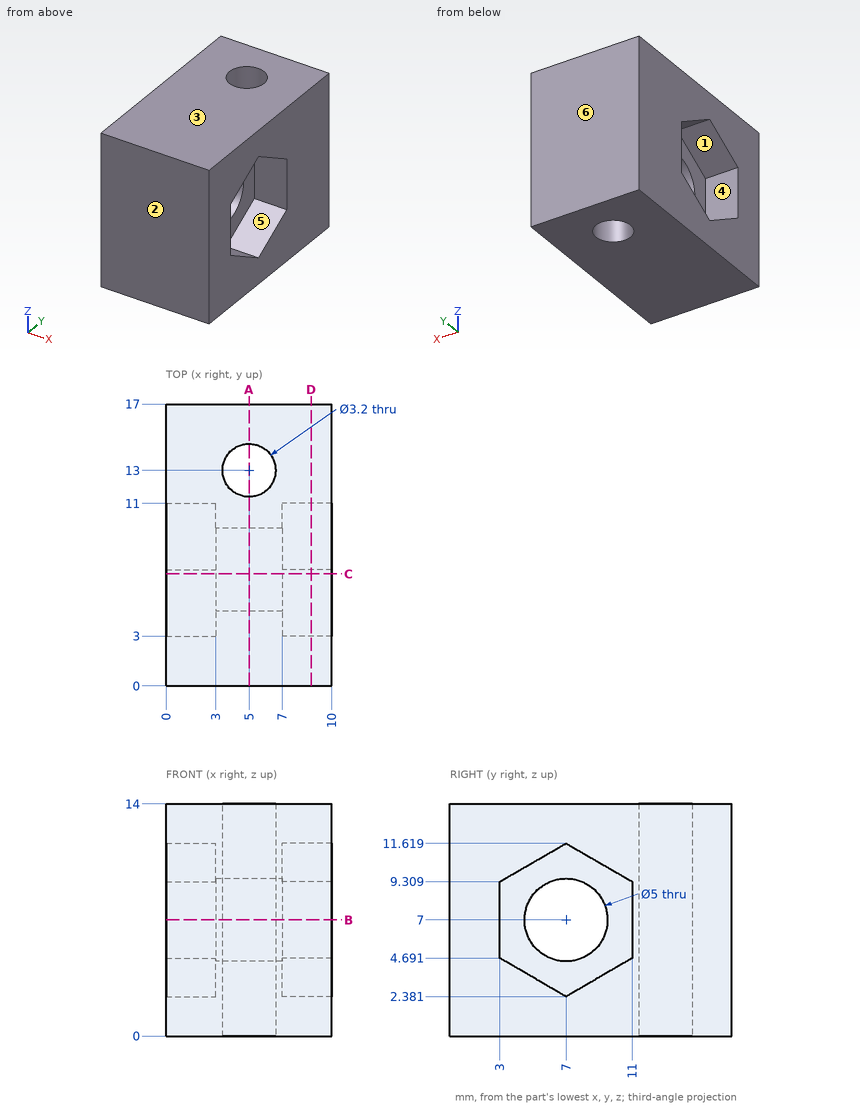
Source: three-view drawing plus pictorial views. Frame: mm from the lowest corner of the part. A direction names the side the tool comes from. Round coordinates to 2 decimals unless told otherwise and drop trailing zeros. Order: outer loops, then holes, each group sorted by start corner. A loop starts at its lowest first (then second) coordinate and runs counter-clockwise, first axis right, second up. Notation, with made-up numbers: M -26,-33 L 29,-33 A31 cw 29,0 Z; hole C -4.75,-26 d4. An arc over 180 degrees is marked long. One line per item, written item: value.
(1) Pin query (flat end, axial travel): P1, Ø6, axis at y = 7, z = 7, coming from the -X side; P2, Ø2.5, axis at y = 6, z = 7, coming from the -X side. Return the tip coordinate at first contact, or that it passes through.
Result sheet:
P1: x = 3
P2: through
(2) Reachability of the marked faces 4, 5 and 6 from +Z, -Z, +X, -X, +Y, -Y: full face, straight path, thin tool, end or side. Return the list, or none.
Result sheet:
face 4: -X
face 5: +X
face 6: +Z, -Z, +X, -X, +Y
(3) Pull-direction query (Y, two-part tool) for the marked faces 1, 2 and 3; classes: pulls with the +Y half, pulls with the -Y half, needs draft (parallel to the pull), parting line crosses it, or undercut.
Result sheet:
face 1: undercut
face 2: pulls with the -Y half
face 3: needs draft
(4) Cut plane A-A (x = 5). Return the cut outline in (y, z).
Result sheet:
outline: M 0,0 L 11.4,0 L 11.4,14 L 0,14 Z; M 14.6,0 L 17,0 L 17,14 L 14.6,14 Z; hole C 7,7 d5
(5) Line query: probe 1 along Y at (x, z) = (5, 8.75) (1 decimal); probe 2 along Y at (x, z) = (5, 11.25); probe 3 along Y at (x, z) = (5, 7.25). Output: solid intervals per line, ascending. Write a range as [from, to].
Result sheet:
probe 1: [0, 5.2], [8.8, 11.4], [14.6, 17]
probe 2: [0, 11.4], [14.6, 17]
probe 3: [0, 4.51], [9.49, 11.4], [14.6, 17]
(6) Cut plane D-D (x = 8.75). Return the cut outline in (y, z).
Result sheet:
outline: M 0,0 L 17,0 L 17,14 L 0,14 Z; hole M 3,4.69 L 7,2.38 L 11,4.69 L 11,9.31 L 7,11.62 L 3,9.31 Z
(7) Cut plane C-C (y = 6.75). Return the cut outline in (x, z) (1 decimal).
Result sheet:
outline: M 0,0 L 10,0 L 10,2.5 L 7,2.5 L 7,4.5 L 3,4.5 L 3,2.5 L 0,2.5 Z; M 0,11.5 L 3,11.5 L 3,9.5 L 7,9.5 L 7,11.5 L 10,11.5 L 10,14 L 0,14 Z
(8) Cut plane B-B (z = 7). Return the cut outline in (x, y).
Result sheet:
outline: M 0,0 L 10,0 L 10,3 L 7,3 L 7,4.5 L 3,4.5 L 3,3 L 0,3 Z; M 0,11 L 3,11 L 3,9.5 L 7,9.5 L 7,11 L 10,11 L 10,17 L 0,17 Z; hole C 5,13 d3.2
